Autodesk Inventor part; units mm, degrees
ref_plane "YZ Plane" through (0, 0, 0) normal (1, 0, 0) x (0, 1, 0)
ref_plane "XZ Plane" through (0, 0, 0) normal (0, 1, 0) x (-1, 0, 0)
ref_plane "XY Plane" through (0, 0, 0) normal (0, 0, 1) x (1, 0, 0)
sketch "Esquisse1" plane through (0, 0, 0) normal (0, 1, 0) x (-1, 0, 0)
  line L0 (4.4286, 5.3714) -> (-11.5714, 5.3714)
  line L1 (-11.5714, 5.3714) -> (-11.5714, -10.6286)
  line L2 (-11.5714, -10.6286) -> (4.4286, -10.6286)
  line L3 (4.4286, -10.6286) -> (4.4286, 5.3714)
  point P0 (0, 0)
  dimension "d0" = 16
  dimension "d1" = 16
extrude "Extrusion1" add sketch "Esquisse1" along normal blind 13
sketch "Esquisse2" plane through (0, 0, 0) normal (0, -1, 0) x (1, 0, 0)
  circle A0 centre (3.5714, -2.6286) radius 4
  line L0 (-4.4286, 5.3714) -> (11.5714, 5.3714)
  line L1 (11.5714, 5.3714) -> (11.5714, -10.6286)
  point P0 (0, 0)
  dimension "d4" = 8
  dimension "d5" = 8
  dimension "d6" = 8
extrude "Extrusion2" cut sketch "Esquisse2" against normal blind 12
sketch "Esquisse3" plane through (3.5714, 12, -2.6286) normal (0, -1, 0) x (1, 0, 0)
  circle A0 centre (0, 0) radius 2.75
  line L0 (8, -8) -> (-8, -8)
  line L1 (8, 8) -> (8, -8)
  point P0 (-3.5714, 2.6286)
  dimension "d9" = 5.5
  dimension "d10" = 8
  dimension "d11" = 8
extrude "Extrusion3" cut sketch "Esquisse3" against normal through all
sketch "Esquisse4" plane through (0, 0, 0) normal (0, -1, 0) x (1, 0, 0)
  circle A0 centre (8.5714, 2.3714) radius 1.5
  circle A1 centre (-1.4286, 2.3714) radius 1.5
  circle A2 centre (-1.4286, -7.6286) radius 1.5
  circle A3 centre (8.5714, -7.6286) radius 1.5
  line L0 (-4.4286, -10.6286) -> (-4.4286, 5.3714)
  line L1 (-4.4286, 5.3714) -> (11.5714, 5.3714)
  line L2 (11.5714, 5.3714) -> (11.5714, -10.6286)
  line L3 (11.5714, -10.6286) -> (-4.4286, -10.6286)
  point P0 (0, 0)
  dimension "d14" = 3
  dimension "d15" = 3
  dimension "d16" = 3
  dimension "d17" = 3
  dimension "d19" = 3
  dimension "d20" = 3
  dimension "d21" = 3
  dimension "d22" = 3
  dimension "d23" = 3
  dimension "d24" = 3
  dimension "d25" = 3
  dimension "d26" = 3
extrude "Extrusion4" cut sketch "Esquisse4" against normal through all contours A0 | A1 | A2 | A3
sketch "Esquisse6" plane through (11.5714, 0, 5.3714) normal (1, 0, 0) x (0, 0, -1)
  line L0 (6.5, 8) -> (9.5, 8)
  line L1 (9.5, 8) -> (9.5, 5)
  line L2 (9.5, 5) -> (6.5, 5)
  line L3 (6.5, 5) -> (6.5, 8)
  line L4 (0, 0) -> (0, 13)
  line L5 (0, 13) -> (16, 13)
  point P0 (5.3714, 0)
  dimension "d29" = 3
  dimension "d30" = 3
  dimension "d31" = 6.5
  dimension "d32" = 5
extrude "Extrusion5" add sketch "Esquisse6" along normal blind 3
sketch "Esquisse7" plane through (14.5714, 0, 5.3714) normal (1, 0, 0) x (0, 0, -1)
  line L0 (5.5, 9) -> (10.5, 9)
  line L1 (10.5, 9) -> (10.5, 4)
  line L2 (10.5, 4) -> (5.5, 4)
  line L3 (5.5, 4) -> (5.5, 9)
  line L4 (0, 13) -> (16, 13)
  line L5 (0, 0) -> (0, 13)
  point P0 (5.3714, 0)
  dimension "d35" = 5
  dimension "d36" = 5
  dimension "d37" = 4
  dimension "d38" = 5.5
extrude "Extrusion6" add sketch "Esquisse7" along normal blind 3
sketch "Esquisse8" plane through (-4.4286, 0, -10.6286) normal (-1, 0, 0) x (0, 0, 1)
  line L0 (0, 0) -> (0, 13)
  line L1 (0, 13) -> (16, 13)
  line L2 (16, 13) -> (16, 0)
  line L3 (16, 0) -> (0, 0)
  line L4 (0, 0) -> (0, 13)
  point P0 (10.6286, 0)
extrude "Extrusion7" add sketch "Esquisse8" along normal blind 7
sketch "Esquisse9" plane through (-11.4286, 0, -10.6286) normal (-1, 0, 0) x (0, 0, 1)
  line L0 (9.5, 8) -> (6.5, 8)
  line L1 (6.5, 8) -> (6.5, 5)
  line L2 (6.5, 5) -> (9.5, 5)
  line L3 (9.5, 5) -> (9.5, 8)
  line L4 (16, 0) -> (16, 13)
  line L5 (16, 13) -> (0, 13)
  point P0 (10.6286, 0)
  dimension "d43" = 6.5
  dimension "d44" = 5
  dimension "d45" = 3
  dimension "d46" = 3
extrude "Extrusion8" add sketch "Esquisse9" along normal blind 3
sketch "Esquisse10" plane through (-14.4286, 0, -10.6286) normal (-1, 0, 0) x (0, 0, 1)
  line L0 (10.5, 9) -> (5.5, 9)
  line L1 (5.5, 9) -> (5.5, 4)
  line L2 (5.5, 4) -> (10.5, 4)
  line L3 (10.5, 4) -> (10.5, 9)
  line L4 (16, 0) -> (16, 13)
  line L5 (0, 0) -> (16, 0)
  point P0 (10.6286, 0)
  dimension "d49" = 5.5
  dimension "d50" = 4
  dimension "d51" = 5
  dimension "d52" = 5
extrude "Extrusion9" add sketch "Esquisse10" along normal blind 3
properties part number "capuchon_roulement_8mm"
Geometry check sheet. Reference: the model listing, model coordinates, mm. A direction names the side the tool comes from. Round coordinates to 2 decimals unless told otherwise and drop trailing zeros. Order: outer loops, then holes, each group sorted by start corner. A loop starts at its lowest first (then second) coordinate and runs counter-clockwise, first axis right, second up. Notation, with made-up numbers: M 31.25,0.25 L 45.25,0.25 A16 cw 45.25,12.25 Z; hole C -39,7.25 d9. An arc over 180 degrees is marked long. Answer in a Markdown table with one row per item. Add a question column.
Item 1: Material ranges on L1, parallel to X at y = 6.75, z = -2.75; L2, parallel to X at y = 11.75, z = -8; L3, parallel to X at y = 8.75, z = -7, recorded low to high. Write a range as [from, to].
Item 2: Sectioned sample at C-C, the plane z = -3.5. Enter the section's corners in (x, y), plus the area to 3 significant figures.
Item 3: Sectioned sample at B-B, the plane x = 5. Enter the section's corners in (y, z).
Item 4: Sectioned sample at D-D, the plane x = 9.5. Enter the section's corners in (y, z).
Item 5: Set-up check for faces 4 (the face through (-13, 7, -4.129)), 5 (the face through (13, 8, -3)), 6 (the face through (16, 9, -3)), 7 (the face through (-16, 4, -3)): record each of +Z, -Z, +X, -X, +Y, -Y from which the full face is reachable in a straight line by a thin tool's end or side.
Item 6: Depth check by flat-ended pin: pin 1 Ø1.5 at (y, z) = (2.5, 2.5) entering from -X; pin 2 Ø2.5 at (x, y) = (16, 5.5) entering from +Z; pin 3 Ø2.5 at (x, z) = (13.5, -2) entering from -Y. Enter the tip coordinate at first touch or a pass-through.
Item 7: Draft check along Z on faces 1 (the face through (0.8, 12, -3.5)), 2 (the face through (0, 13, -3)), 3 (the face through (-13, 6, -1.129)). Enter one of: released by +Z, released by -Z, zero draft, split by the parting line, or undercut.
Item 8: Sectioned sample at A-A, the plane y = 7.5. Enter the section's corners in (x, z).
Filled in:
| question | item | result |
|---|---|---|
| 1 | L1 | x = [-17.43, -0.43], [7.57, 17.57] |
| 1 | L2 | x = [-11.43, -2.88], [0.02, 7.12], [10.02, 11.57] |
| 1 | L3 | x = [-11.43, -2.79], [-0.07, 7.21], [9.93, 11.57] |
| 2 | outline | M -17.43,4 L -14.43,4 L -14.43,5 L -11.43,5 L -11.43,0 L -0.33,0 L -0.33,12 L 0.96,12 L 0.96,13 L -11.43,13 L -11.43,8 L -14.43,8 L -14.43,9 L -17.43,9 Z; M 6.18,12 L 7.48,12 L 7.48,0 L 11.57,0 L 11.57,5 L 14.57,5 L 14.57,4 L 17.57,4 L 17.57,9 L 14.57,9 L 14.57,8 L 11.57,8 L 11.57,13 L 6.18,13 Z |
| 2 | area | 248 mm² |
| 3 | outline | M 0,-10.63 L 13,-10.63 L 13,-4.98 L 12,-4.98 L 12,-6.36 L 0,-6.36 Z; M 0,1.11 L 12,1.11 L 12,-0.28 L 13,-0.28 L 13,5.37 L 0,5.37 Z |
| 4 | outline | M 0,-10.63 L 13,-10.63 L 13,-8.81 L 0,-8.81 Z; M 0,-6.45 L 13,-6.45 L 13,1.19 L 0,1.19 Z; M 0,3.55 L 13,3.55 L 13,5.37 L 0,5.37 Z |
| 5 | face 4 | -Z, +Y, -Y |
| 5 | face 5 | +Z, -Z, +Y |
| 5 | face 6 | +Z, -Z, +X, +Y |
| 5 | face 7 | +Z, -Z, -X, -Y |
| 6 | pin 1 | stops at x = -11.43 |
| 6 | pin 2 | stops at z = -0.13 |
| 6 | pin 3 | stops at y = 4 |
| 7 | face 1 | undercut |
| 7 | face 2 | zero draft |
| 7 | face 3 | released by +Z |
| 8 | outline | M -17.43,-5.13 L -14.43,-5.13 L -14.43,-4.13 L -11.43,-4.13 L -11.43,-10.63 L 11.57,-10.63 L 11.57,-4.13 L 14.57,-4.13 L 14.57,-5.13 L 17.57,-5.13 L 17.57,-0.13 L 14.57,-0.13 L 14.57,-1.13 L 11.57,-1.13 L 11.57,5.37 L -11.43,5.37 L -11.43,-1.13 L -14.43,-1.13 L -14.43,-0.13 L -17.43,-0.13 Z; hole C -1.43,-7.63 d3; hole C -1.43,2.37 d3; hole C 3.57,-2.63 d8; hole C 8.57,-7.63 d3; hole C 8.57,2.37 d3 |
